Geometry: final body of the model. Coordinates: model frame, mm. Face numbers are marked on the shaded views. A direction names the side the tool comes from. Give positions to 0.01 mm unless a question says otherwise; leave off trailing zeros. Write each loop counter-clockwise with the first axis right and the second up, starting at its lowest first coordinate (ties: lowest second). Pieces come first, ordered by that corner, then holes. Notation, with made-up numbers: M -23,-15.5 L 35,-15.5 A22 cw 35,16.5 Z; hole C 31,-20 d11. An arc over 180 degrees is marked long. Answer as a JSON object with one key per item and string values.
Autodesk Inventor part; units mm, degrees
ref_plane "YZ Plane" through (0, 0, 0) normal (1, 0, 0) x (0, 1, 0)
ref_plane "XZ Plane" through (0, 0, 0) normal (0, 1, 0) x (-1, 0, 0)
ref_plane "XY Plane" through (0, 0, 0) normal (0, 0, 1) x (1, 0, 0)
sketch "Sketch1" plane through (0, 0, 0) normal (1, 0, 0) x (0, 1, 0)
  circle A0 centre (0, 0) radius 88.9
  dimension "d0" = 177.8
extrude "Extrusion1" add sketch "Sketch1" along normal blind 50.8
sketch "Sketch2" plane through (50.8, 0, 0) normal (1, 0, 0) x (0, 0, -1)
  circle A0 centre (0, 0) radius 88.9
  circle A1 centre (0, 0) radius 76.2
  dimension "d3" = 12.7
extrude "Extrusion2" cut sketch "Sketch2" against normal blind 12.7 contours A1
sketch "Sketch4" plane through (0, 0, 0) normal (-1, 0, 0) x (0, 0, 1)
  circle A0 centre (0, 0) radius 76.2
extrude "Extrusion3" cut sketch "Sketch4" against normal blind 12.7
sketch "Sketch5" plane through (38.1, 0, 0) normal (1, 0, 0) x (0, 0, -1)
  line L0 (0, 0) -> (0, 12.7)
  line L1 (0, 12.7) -> (10.9985, 6.35)
  line L2 (10.9985, 6.35) -> (10.9985, -6.35)
  line L3 (10.9985, -6.35) -> (0, -12.7)
  line L4 (0, -12.7) -> (-10.9985, -6.35)
  line L5 (-10.9985, -6.35) -> (-10.9985, 6.35)
  line L6 (-10.9985, 6.35) -> (0, 12.7)
  dimension "d8" = 12.7
extrude "Extrusion4" cut sketch "Sketch5" against normal blind 127
properties part number "WheelV1"
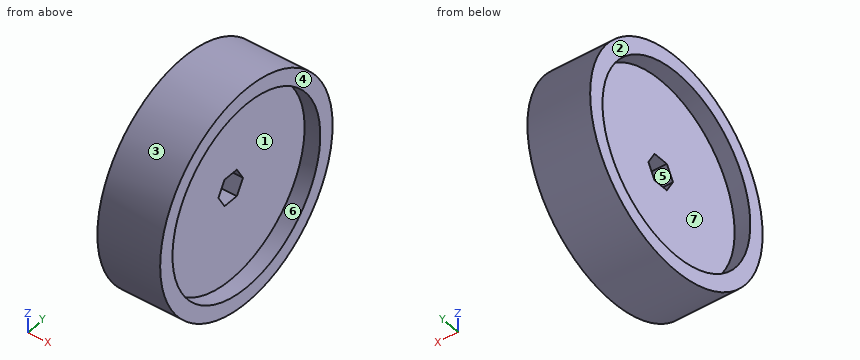
1) Cut plane A-A on y = 0. Return loops of the section in (x, z), and give its area (3 significant figures).
Geometry check:
{"outline": "M 0,-88.9 L 50.8,-88.9 L 50.8,-76.2 L 38.1,-76.2 L 38.1,-11 L 12.7,-11 L 12.7,-76.2 L 0,-76.2 Z; M 0,76.2 L 12.7,76.2 L 12.7,11 L 38.1,11 L 38.1,76.2 L 50.8,76.2 L 50.8,88.9 L 0,88.9 Z", "area": "4,600 mm2"}
2) Cut plane C-C on z = -46. Return loops of the section in (x, y).
Geometry check:
{"outline": "M 0,-76.07 L 50.8,-76.07 L 50.8,-60.75 L 38.1,-60.75 L 38.1,60.75 L 50.8,60.75 L 50.8,76.07 L 0,76.07 L 0,60.75 L 12.7,60.75 L 12.7,-60.75 L 0,-60.75 Z"}
3) Pull-direction query (Z, two-part tool) for the marked faces 1, 2 and 3; classes: pulls with the +Z half, pulls with the -Z half, needs draft (parallel to the pull), parting line crosses it, or undercut.
Geometry check:
{"face 1": "undercut", "face 2": "needs draft", "face 3": "parting line crosses it"}
4) Line query: line 1 (X direction, y = -11, z = 7); line 2 (Z direction, x = 6, y = 44); line 3 (Z direction, x = 3, y = 32.5). Output: solid intervals per line, ascending. Write a range as from..to.
Geometry check:
{"line 1": "x = 12.7..38.1", "line 2": "z = -77.25..-62.21, 62.21..77.25", "line 3": "z = -82.75..-68.92, 68.92..82.75"}
5) Set-up query: the marked faces 4, 5, 6 and 7. Return all of +Z, -Z, +X, -X, +Y, -Y with unobstructed straight access to the full face (end or side cutting, diameter ignored); none if empty.
Geometry check:
{"face 4": "+Z, -Z, +X, +Y, -Y", "face 5": "+X, -X", "face 6": "+X", "face 7": "-X"}
6) Cut plane B-B on x = 21.5. Return loops of the section in (y, z), and give its area (3 significant figures).
Geometry check:
{"outline": "C 0,0 d177.8; hole M -12.7,0 L -6.35,-11 L 6.35,-11 L 12.7,0 L 6.35,11 L -6.35,11 Z", "area": "24,400 mm2"}
7) Contact query for flat-ended pins moving along their axis: P1, Ø8, axis at x = 18.5, z = -5, coming from the +Y side; P2, Ø2, axis at x = 7.5, y = -46, coming from the +Z side; P3, Ø10, axis at x = 6, z = 38.5, coming from the -Y side. Output: stop coordinate, or through.
Geometry check:
{"P1": "stops at y = 88.89", "P2": "stops at z = 76.67", "P3": "stops at y = -82.35"}
8) Cut plane D-D on y = 67. Return loops of the section in (x, z).
Geometry check:
{"outline": "M 0,-58.43 L 50.8,-58.43 L 50.8,-36.3 L 38.1,-36.3 L 38.1,36.3 L 50.8,36.3 L 50.8,58.43 L 0,58.43 L 0,36.3 L 12.7,36.3 L 12.7,-36.3 L 0,-36.3 Z"}
